from build123d import *

# Parameters (mm, degrees)
F3_R     = 14.8532695911
F3_W     = 21
F3_H     = 11
F4_DEPTH = 77
F5_R     = 14.8532695911
F6_DEPTH = 3
F7_R     = 0.5


with BuildPart() as f4:
    # F3 (on Front) → F4 (new body)
    with BuildSketch(Plane.XZ):
        Circle(F3_R)
        Rectangle(F3_W, F3_H, mode=Mode.SUBTRACT)
    extrude(amount=-F4_DEPTH)

    # F5 (on face) → F6 (join)
    with BuildSketch(Plane(origin=(0, 77, 0), x_dir=(-1, 0, 0), z_dir=(0, 1, 0))):
        Circle(F5_R)
    extrude(amount=F6_DEPTH)

    # F7
    f7_edges = [f4.edges().sort_by_distance(p)[0] for p in [
        (-10.5, 77, 0),
        (0, 77, -5.5),
        (10.5, 77, 0),
        (0, 77, 5.5),
        (-10.5, 38.5, -5.5),
        (-10.5, 38.5, 5.5),
        (10.5, 38.5, 5.5),
        (10.5, 38.5, -5.5),
    ]]
    fillet(f7_edges, radius=F7_R)


solid = f4.part
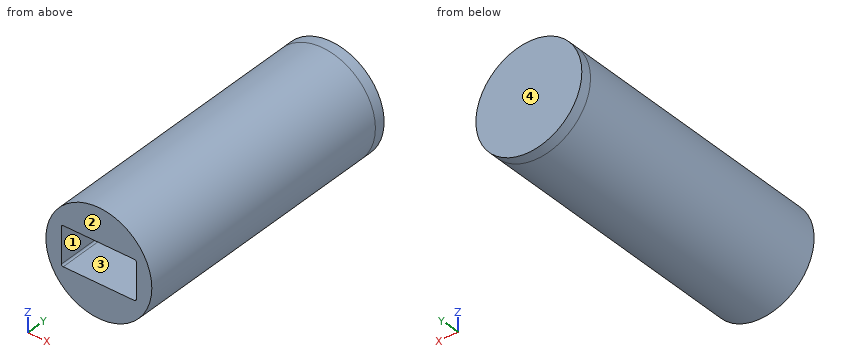
For this review, take the finished solid that the model builds, in its own axes (mm). Face numbers are marked on the shaded views. A direction names the side the tool comes from. Round coordinates to 2 decimals unless told otherwise and drop trailing zeros. Loops run counter-clockwise (first coordinate to the right, second up) from the corner with the lowest first, then second, coordinate; pieces in that order, holes last. Notation, with made-up numbers: (48, 66.25) - (89, 66.25) arc R4 cw to (89, 71.25) - close; hole circle Ø11 at (-25, 69). An arc over 180 degrees is marked (long way). Put each result on its own line as item: value. Start each with the question number.
1. Consider section C-C on x = 0. State the section outline as (y, z) points, plus the area to 3 significant figures.
2. Consider section B-B on z = 0. State the section outline as (x, y) points, plus the area to 3 significant figures.
3. Consider section A-A on y = 47.5. State the section outline as (x, z) points, plus the area to 3 significant figures.
4. For the marked faces 3 and 4, list the 3-axis set-ups (+Z, -Z, +X, -X, +Y, -Y) from which the entire face can be reached by the end or side of a thin tool; tool diameter is ignored.
5. Mouldability with a two-part tool opening along Z and no side actions: class the marked faces 1 and 2 as +Z half, -Z half, draft (parallel to the pull), parting line (faces both ways), or undercut.
6. For probe 1 along Z at (x, y) = (0, 52); probe 2 along Y at (x, z) = (0.25, 0.75); probe 3 along Z at (x, y) = (3.5, 64.5), list the stretches that pass through material, from the lowest coordinate up. Write a range as [from, to].
7. Consider section D-D on z = 7.5. State the section outline as (x, y) points.
8. Insertion check: P1, Ø5, axis at x = 4.5, z = -1.5, coming from the -Y side; P2, Ø5, axis at x = -6, y = 44.5, coming from the +Z side (3 decimals); P3, Ø3, axis at x = -4.5, y = 11, coming from the +Z side. Each pin has a flat end and moves straight along its axis. Give the tip position at first contact, or say it passes through.
Result sheet:
1. outline: (0, -14.85) - (80, -14.85) - (80, 14.85) - (0, 14.85) - (0, 5.5) - (76.5, 5.5) arc R0.5 cw to (77, 5) - (77, -5) arc R0.5 cw to (76.5, -5.5) - (0, -5.5) - close
1. area: 1,530 mm^2
2. outline: (-14.85, 0) - (-10.5, 0) - (-10.5, 76.5) arc R0.5 cw to (-10, 77) - (10, 77) arc R0.5 cw to (10.5, 76.5) - (10.5, 0) - (14.85, 0) - (14.85, 80) - (-14.85, 80) - close
2. area: 760 mm^2
3. outline: circle Ø29.71 at (0, 0); hole (-10.5, -5) arc R0.5 ccw to (-10, -5.5) - (10, -5.5) arc R0.5 ccw to (10.5, -5) - (10.5, 5) arc R0.5 ccw to (10, 5.5) - (-10, 5.5) arc R0.5 ccw to (-10.5, 5) - close
3. area: 462 mm^2
4. face 3: -Y
4. face 4: +Z, -Z, +X, -X, +Y
5. face 1: undercut
5. face 2: draft
6. probe 1: [-14.85, -5.5], [5.5, 14.85]
6. probe 2: [77, 80]
6. probe 3: [-14.44, -5.5], [5.5, 14.44]
7. outline: (-12.82, 0) - (12.82, 0) - (12.82, 80) - (-12.82, 80) - close
8. P1: y = 77
8. P2: z = 14.435
8. P3: z = 14.55
